```python
from build123d import *

# Parameters (mm, degrees)
F1_DEPTH  = 60
F3_DEPTH  = 25
F4_W      = 7.5
F4_H      = 10
F5_DEPTH  = 70
F6_R      = 34.99999
F7_R      = 5
F8_R      = 15
F9_DEPTH  = 50
F11_DEPTH = 90
F13_DEPTH = 45
F14_R     = 5


# Not quite as in the source:
# - a fillet or chamfer is up to 0.001 mm smaller than in the source, because OpenCascade refuses the exact size
# - a pattern or mirror of a feature is missing from the dataset's text; its kind, count and spacing are read off the source's solid


with BuildPart() as f1:
    # F0 (on Front) → F1 (new body, symmetric)
    with BuildSketch(Plane.XZ):
        Polygon((-180, 0), (0, 0), (180, 0), (180, 50), (90.5, 50), (72.5, 90), (0, 90), (-72.5, 90), (-90.5, 50), (-180, 50), align=None)
    extrude(amount=F1_DEPTH, both=True)

    # F2 (on face) → F3 (cut)
    with BuildSketch(Plane.XZ.offset(60)):
        Polygon((-95, 40), (-90.5, 50), (-180, 50), (-180, 40), align=None)
        Polygon((180, 50), (90.5, 50), (95, 40), (180, 40), align=None)
    f3 = extrude(amount=-F3_DEPTH, mode=Mode.SUBTRACT)

    # F3_copies: F3 across plane
    add(f3.mirror(Plane.ZX), mode=Mode.SUBTRACT)

    # F4 (on face) → F5 (cut)
    with BuildSketch(Plane.XZ.offset(35)):
        with Locations((-176.25, 45)):
            Rectangle(F4_W, F4_H)
        with Locations((176.25, 45)):
            Rectangle(F4_W, F4_H)
    extrude(amount=-F5_DEPTH, mode=Mode.SUBTRACT)

    # F6 (radius 35 in the source; OpenCascade refuses exactly that, so slightly less here)
    f6_edges = [f1.edges().sort_by_distance(p)[0] for p in [
        (172.5, -35, 45),
        (172.5, 35, 45),
        (-172.5, -35, 45),
        (-172.5, 35, 45),
    ]]
    fillet(f6_edges, radius=F6_R)

    # F7
    f7_edges = [f1.edges().sort_by_distance(p)[0] for p in [
        (116.250005, -35, 40),
        (95, -47.5, 40),
        (-116.250005, -35, 40),
        (-95, -47.5, 40),
        (-162.24874, -24.74874, 40),
        (-172.5, 0, 40),
        (-162.24874, 24.74874, 40),
        (-116.250005, 35, 40),
        (-95, 47.5, 40),
        (116.250005, 35, 40),
        (162.24874, 24.74874, 40),
        (95, 47.5, 40),
        (172.5, 0, 40),
        (162.24874, -24.74874, 40),
    ]]
    fillet(f7_edges, radius=F7_R)

    # F8 (on face) → F9 (cut)
    with BuildSketch(Plane.XY.offset(50)):
        with Locations((-137.5, 0)):
            Circle(F8_R)
        with Locations((137.5, 0)):
            Circle(F8_R)
    extrude(amount=-F9_DEPTH, mode=Mode.SUBTRACT)

    # F10 (on face) → F11 (cut)
    with BuildSketch(Plane.XY.offset(90)):
        with BuildLine():
            ThreePointArc((0, 30), (-8.8388347648, 26.3388347648), (-12.5, 17.5))
            Line((-12.5, 17.5), (-12.5, -17.5))
            ThreePointArc((-12.5, -17.5), (-8.8388347648, -26.3388347648), (0, -30))
            ThreePointArc((0, -30), (8.8388347648, -26.3388347648), (12.5, -17.5))
            Line((12.5, -17.5), (12.5, 17.5))
            ThreePointArc((12.5, 17.5), (8.8388347648, 26.3388347648), (0, 30))
        make_face()
    extrude(amount=-F11_DEPTH, mode=Mode.SUBTRACT)

    # F12 (on Front) → F13 (cut, symmetric)
    with BuildSketch(Plane.XZ):
        Polygon((-62.5, 75), (-96.25, 0), (0, 0), (96.25, 0), (62.5, 75), (0, 75), align=None)
    extrude(amount=F13_DEPTH, both=True, mode=Mode.SUBTRACT)

    # F14
    f14_edges = [f1.edges().sort_by_distance(p)[0] for p in [
        (79.375, -45, 37.5),
        (0, -45, 75),
        (62.5, 0, 75),
        (-62.5, 0, 75),
        (-79.375, -45, 37.5),
        (-79.375, 45, 37.5),
        (0, 45, 75),
        (79.375, 45, 37.5),
    ]]
    fillet(f14_edges, radius=F14_R)


solid = f1.part
```
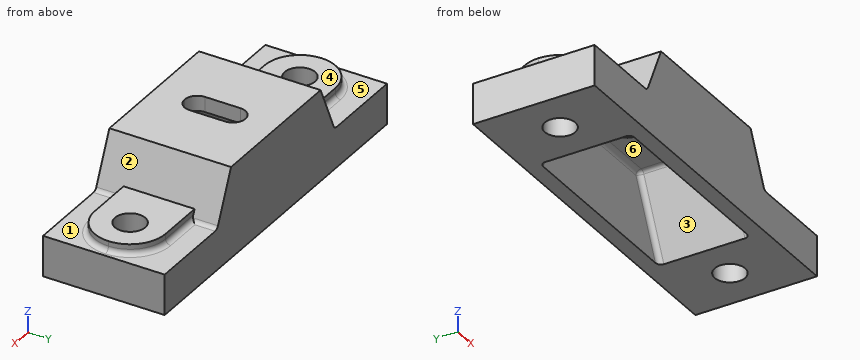
The listing builds one solid part. Answer for the finished solid, in the listing's coordinates (mm). Face numbers are marked on the shaded views. A direction names the side the tool comes from. Coordinates: 2 decimals unless noted, no trailing zeros. Loops run counter-clockwise (first coordinate to the right, second up) from the corner with the lowest first, then second, coordinate; pieces in that order, holes last. Notation, with made-up numbers: (-12, -17.75) - (43, -17.75) arc R33 ccw to (43, 13.25) - close; hole circle Ø10 at (-25, 67). An arc over 180 degrees is marked (long way). Write item = value, one per line.
1) Find the intervals of material crossed by line 1 along Y through (x, z) = (137, 15); line 2 along Y through (x, z) = (-16.5, 23.5); line 3 along Z through (x, y) = (36.5, -23.5), in increasing order.
Responses:
line_1 = -60 to -14.99, 14.99 to 60
line_2 = -60 to -45, 45 to 60
line_3 = 75 to 90
2) Section A-A (z = 82) is taken. Determine the outline of the cut face in (x, y), plus the area to 3 significant figures.
Responses:
outline = (-76.1, -60) - (76.1, -60) - (76.1, 60) - (-76.1, 60) - close; hole (-12.5, -17.5) arc R12.5 ccw to (12.5, -17.5) - (12.5, 17.5) arc R12.5 ccw to (-12.5, 17.5) - close
area = 16,900 mm^2
3) Which of the six approach directions +Z, -Z, +X, -X, +Y, -Y give full straight-line access (tool end or side, diameter ignored) to the marked faces 4, 5 and 6?
Responses:
face_4 = +Z, -X, +Y, -Y
face_5 = +Z, -X, +Y
face_6 = -Z
4) Section D-D (z = 17) is taken. Count the separate pieces of the cut face and the enclosed holes in it, plus the area to 3 significant figures.
Responses:
separate_pieces = 1
enclosed_holes = 3
area = 25,900 mm^2
5) Each of these flat-tipped pins is pushed along its axis until it touches: P1, Ø1.5, axis at x = 70.5, y = 29, coming from the -Z side; P2, Ø1.5, axis at x = 106, z = 48, coming from the -Y side; P3, Ø4, axis at x = 94, y = -6.5, coming from the -Z side. Where does it stop, or does it pass through?
Responses:
P1 = 55.56
P2 = -35
P3 = 0.56
6) Section C-C (x = 40) is taken. Determine the outline of the cut face in (y, z), plus the area to 3 significant figures.
Responses:
outline = (-60, 0) - (-45, 0) - (-45, 70) arc R5 cw to (-40, 75) - (40, 75) arc R5 cw to (45, 70) - (45, 0) - (60, 0) - (60, 90) - (-60, 90) - close
area = 4,060 mm^2
7) Determine the mould class of the marked faces 1, 2 and 3 for opening direction X: pulls with the +X half, pulls with the -X half, needs draft (parallel to the pull), parting line crosses it, or undercut.
Responses:
face_1 = needs draft
face_2 = pulls with the +X half
face_3 = undercut
8) Section B-B (x = -7) is taken. Determine the outline of the cut face in (y, z), plus the area to 3 significant figures.
Responses:
outline = (-60, 0) - (-45, 0) - (-45, 70) arc R5 cw to (-40, 75) - (-27.86, 75) - (-27.86, 90) - (-60, 90) - close; (27.86, 75) - (40, 75) arc R5 cw to (45, 70) - (45, 0) - (60, 0) - (60, 90) - (27.86, 90) - close
area = 3,230 mm^2
